```python
from build123d import *

# Parameters (mm, degrees)
F0_R     = 35
F1_DEPTH = 40
F2_R     = 35
F2_R_2   = 31.25
F3_DEPTH = 20
F2_R_3   = 29
F4_DEPTH = 40


with BuildPart() as f1:
    # F0 (on Top) → F1 (new body)
    with BuildSketch(Plane.XY):
        Circle(F0_R)
    extrude(amount=F1_DEPTH)

    # F2 (on face) → F3 (cut)
    with BuildSketch(Plane.XY.offset(40)):
        Circle(F2_R)
        Circle(F2_R_2, mode=Mode.SUBTRACT)
    extrude(amount=-F3_DEPTH, mode=Mode.SUBTRACT)

    # F2 (on face) → F4 (cut)
    with BuildSketch(Plane.XY.offset(40)):
        Circle(F2_R_3)
    extrude(amount=-F4_DEPTH, mode=Mode.SUBTRACT)


solid = f1.part
```
Verification items for the finished model (mm, model axes). A direction names the side the tool comes from. Round coordinates to 2 decimals unless told otherwise and drop trailing zeros. Loops run counter-clockwise (first coordinate to the right, second up) from the corner with the lowest first, then second, coordinate; pieces in that order, holes last. Notation, with made-up numbers: (53, -12) -> (84, -12) arc R14 cw to (84, 13) -> close; hole circle Ø10 at (10.25, -40). An arc over 180 degrees is marked (long way). Answer as a JSON object with one key per item and string values.
Q1. Go/stop test with flat-tipped pins: P1, Ø6, axis at y = 21, z = 23.5, coming from the -X side; P2, Ø5, axis at x = 24.5, z = 4.5, coming from the -Y side; P3, Ø10, axis at y = 9, z = 35.5, coming from the -X side. Record where each tip stops, or that it passes through.
Data:
{"P1": "stops at x = -25.55", "P2": "stops at y = -27.22", "P3": "stops at x = -30.99"}
Q2. Access from +Z, -Z, +X, -X, +Y, -Y to the whole of each face (thin tool, end or side, straight path). Record for faces 4 (the flat face through (28, -9, 40)), 5 (the flat face through (-13, 29, 20)).
Data:
{"face 4": "+Z, +X, -X, +Y, -Y", "face 5": "+Z"}
Q3. Scan lines: line 1 (Y direction, x = 0, z = 16); line 2 (Y direction, x = 0, z = 27); line 3 (X direction, y = 20, z = 33.5). Record each from-to range of solid material in increasing order. Write a range as from..to.
Data:
{"line 1": "y = -35..-29, 29..35", "line 2": "y = -31.25..-29, 29..31.25", "line 3": "x = -24.01..-21, 21..24.01"}
Q4. Draft check along Y on faces 1 (the flat face through (-13.1, 26.1, 0)), 2 (the cylindrical face through (-28, -21, 10)), 3 (the cylindrical face through (13.38, -25.73, 20.28)). Enter one of: pulls with the +Y half, pulls with the -Y half, needs draft (parallel to the pull), parting line crosses it, or undercut.
Data:
{"face 1": "needs draft", "face 2": "parting line crosses it", "face 3": "undercut"}
Q5. Section check A-A (y = 0). Record the boundary of the cut face in (x, z), then the cut area to 3 significant figures.
Data:
{"outline": "(-35, 0) -> (-29, 0) -> (-29, 40) -> (-31.25, 40) -> (-31.25, 20) -> (-35, 20) -> close; (29, 0) -> (35, 0) -> (35, 20) -> (31.25, 20) -> (31.25, 40) -> (29, 40) -> close", "area": "330 mm2"}
Q6. Section check D-D (z = 37.5). Record the boundary of the cut face in (x, y).
Data:
{"outline": "circle Ø62.5 at (0, 0); hole circle Ø58 at (0, 0)"}
Q7. Section check C-C (z = 16). Record the boundary of the cut face in (x, y).
Data:
{"outline": "circle Ø70 at (0, 0); hole circle Ø58 at (0, 0)"}
